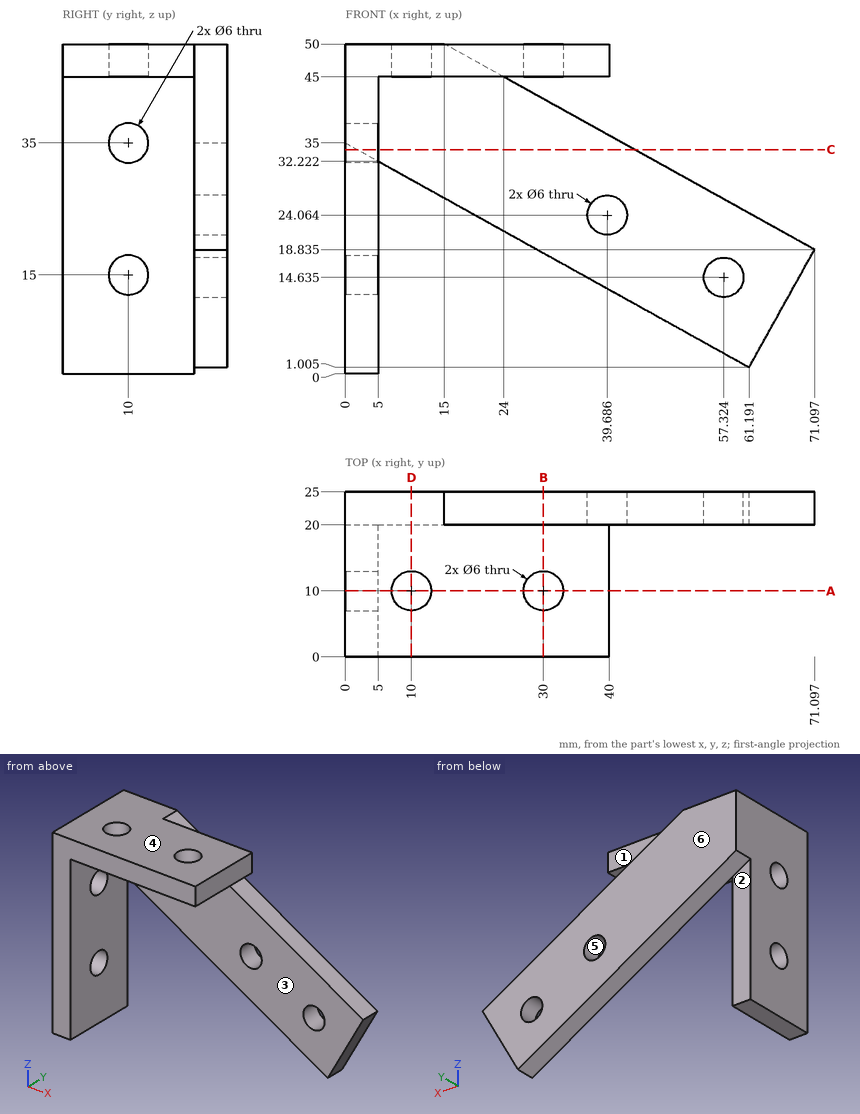
The figure shows three views and two pictorial views of one solid part (mm, origin at its lowest corner). Answer the questions. A direction names the side the tool comes from. Coordinates: 2 decimals unless noted, no trailing zeros. Loops run counter-clockwise (first coordinate to the right, second up) from the corner with the lowest first, then second, coordinate; pieces in that order, holes last. Notation, with made-up numbers: (-13, 25) - (43, 25) arc R6 ccw to (43, 31) - close; hole circle Ø9 at (28, 89.25). An arc over 180 degrees is marked (long way). Use a Markdown table: item, result. Add a question column.
1) For the marked faces 1, 2 and 3, determine the directions among +Z, -Z, +X, -X, +Y, -Y from which every point of the face is accessible in a straight line to the end or side of a thin tool.
2) The part is cut by section D-D, the plane x = 10. Give the vertices of the cut face in (y, z) (1 decimal).
3) The part is cut by section A-A, the plane y = 10. Give the vertices of the cut face in (x, z), and give its area (3 significant figures).
4) Given pin 1 (5 mm diameter, centred on y = 15.5, z = 26, fed in from +X); pin 2 (2.5 mm diameter, centred on y = 9, z = 48, fed in from +X); pin 3 (6 mm diameter, centred on x = 18, y = 14.5, fed in from -Z); pin 4 (8 mm diameter, centred on x = 30, y = 10, fed in from +Z), each flat-ended and moving along its own axis, determine where each tip first touches the part or whether it passes through.
5) The part is cut by section C-C, the plane z = 34. Give the vertices of the cut face in (x, y).
6) The part is cut by section B-B, the plane x = 30. Give the vertices of the cut face in (y, z).
7) The mould has two halves that part along Z. Classify the marked faces 4, 5 and 6: released by +Z, released by -Z, zero draft, split by the parting line, or undercut.
8) Find the intervals of material crossed by line 1 (Y direction, x = 30, z = 47.5); line 2 (Y direction, x = 10, z = 47.1); line 3 (Y direction, x = 22, z = 26), in increasing order.
Here are the results:
| question | item | result |
|---|---|---|
| 1 | face 1 | +Z, +X, +Y |
| 1 | face 2 | -Z, -X, +Y |
| 1 | face 3 | -Z, +X, -Y |
| 2 | outline | (0, 45) - (7, 45) - (7, 50) - (0, 50) - close; (13, 45) - (20, 45) - (20, 29.4) - (25, 29.4) - (25, 50) - (13, 50) - close |
| 3 | outline | (0, 0) - (5, 0) - (5, 12) - (0, 12) - close; (0, 18) - (5, 18) - (5, 32) - (0, 32) - close; (0, 38) - (5, 38) - (5, 45) - (7, 45) - (7, 50) - (0, 50) - close; (13, 45) - (27, 45) - (27, 50) - (13, 50) - close; (33, 45) - (40, 45) - (40, 50) - (33, 50) - close |
| 3 | area | 305 mm^2 |
| 4 | pin 1 | stops at x = 5 |
| 4 | pin 2 | stops at x = 40 |
| 4 | pin 3 | stops at z = 45 |
| 4 | pin 4 | stops at z = 50 |
| 5 | outline | (0, 0) - (5, 0) - (5, 7.17) - (0, 7.17) - close; (0, 12.83) - (5, 12.83) - (5, 20) - (43.8, 20) - (43.8, 25) - (1.8, 25) - (1.8, 20) - (0, 20) - close |
| 6 | outline | (0, 45) - (7, 45) - (7, 50) - (0, 50) - close; (13, 45) - (20, 45) - (20, 50) - (13, 50) - close; (20, 18.33) - (25, 18.33) - (25, 41.67) - (20, 41.67) - close |
| 7 | face 4 | released by +Z |
| 7 | face 5 | undercut |
| 7 | face 6 | zero draft |
| 8 | line 1 | y = 0 to 7, 13 to 20 |
| 8 | line 2 | y = 0 to 7, 13 to 25 |
| 8 | line 3 | y = 20 to 25 |
